Input: part model. Units: mm. Frame: model coordinates. Coordinates: 2 decimals unless noted, no trailing zeros. Write each loop counter-clockwise with the first axis right and the second up, starting at its lowest first coordinate (ties: lowest second). Pieces come first, ordered by that corner, then holes. Notation, with made-up numbers: (17, 4) -> (67, 4) arc R11 ccw to (67, 13) -> close; hole circle Ø8 at (76, 25). An arc over 180 degrees is marked (long way). One line per question, with ' | ' between items. Start each with the question number.
Autodesk Inventor part; units mm, degrees
ref_plane "YZ Plane" through (0, 0, 0) normal (1, 0, 0) x (0, 1, 0)
ref_plane "XZ Plane" through (0, 0, 0) normal (0, 1, 0) x (-1, 0, 0)
ref_plane "XY Plane" through (0, 0, 0) normal (0, 0, 1) x (1, 0, 0)
sketch "スケッチ1" plane through (0, 0, 0) normal (0, 0, 1) x (1, 0, 0)
  line L0 (7.5, 7.5) -> (-7.5, 7.5)
  line L1 (-7.5, 7.5) -> (-7.5, -7.5)
  line L2 (-7.5, -7.5) -> (7.5, -7.5)
  line L3 (7.5, -7.5) -> (7.5, 7.5)
  line L4 (7.5, 7.5) -> (-7.5, -7.5) construction
  line L5 (-7.5, 7.5) -> (7.5, -7.5) construction
  point P0 (0, 0)
  dimension "d0" = 15
  dimension "d1" = 15
extrude "押し出し1" add sketch "スケッチ1" along normal blind 1000
shell "シェル1" thickness 1 removed faces 2 at (-2.5, 2.5, 0) at (-2.5, 2.5, 1000)
sketch "スケッチ2" plane through (-7.5, -7.5, 0) normal (-1, 0, 0) x (0, 0, 1)
  line L0 (0, 0) -> (0, 15)
  line L1 (0, 15) -> (1000, 15)
  line L2 (1000, 0) -> (1000, 15)
  line L3 (0, 0) -> (1000, 0)
  line L4 (1000, 15) -> (1000, 0)
  line L5 (0, 15) -> (0, 0)
  point P0 (5, 7.5)
  point P1 (15, 7.5)
  point P2 (25, 7.5)
  point P3 (995, 7.5)
  point P4 (985, 7.5)
  point P5 (975, 7.5)
  point P6 (1000, 7.5)
  point P7 (0, 7.5)
  dimension "d5" = 10
  dimension "d6" = 10
  dimension "d9" = 10
  dimension "d10" = 10
  dimension "d18" = 5
  dimension "d19" = 5
hole "穴1" at (-7.5, 0, 5) at (-7.5, 0, 15) at (-7.5, 0, 25) at (-7.5, 0, 995) at (-7.5, 0, 985) at (-7.5, 0, 975) direction (1, 0, 0) diameter 3.2 end through all
properties part number "□15"
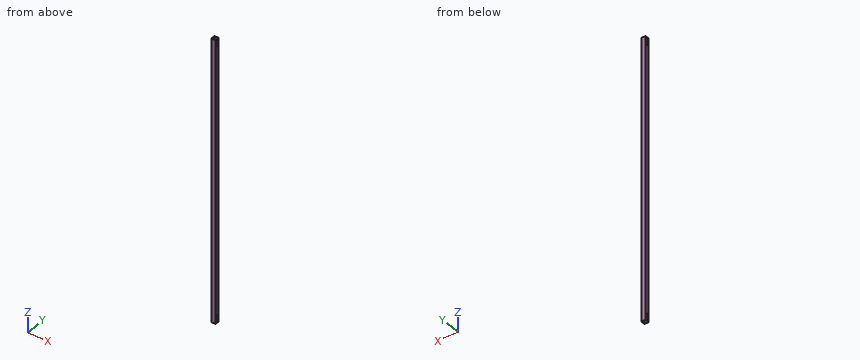
1) Ray query, line 1 (Y direction, x = 6.75, z = 995); line 2 (X direction, y = -1.75, z = 507). Return the intervals inside material, ascending.
2) Section A-A, the plane z = 372. Return loops of the section in (x, y).
3) Section B-B, the plane y = 4.25. Return loops of the section in (x, z), then the cut area to 3 significant figures.
Answer block:
1) line 1: y = -7.5 to -1.6, 1.6 to 7.5 | line 2: x = -7.5 to -6.5, 6.5 to 7.5
2) outline: (-7.5, -7.5) -> (7.5, -7.5) -> (7.5, 7.5) -> (-7.5, 7.5) -> close; hole (-6.5, -6.5) -> (6.5, -6.5) -> (6.5, 6.5) -> (-6.5, 6.5) -> close
3) outline: (-7.5, 0) -> (-6.5, 0) -> (-6.5, 1000) -> (-7.5, 1000) -> close; (6.5, 0) -> (7.5, 0) -> (7.5, 1000) -> (6.5, 1000) -> close | area: 2,000 mm2
